from build123d import *

# Parameters (mm, degrees)
BOSS_EXTRUDE1_DEPTH                   = 6.35
FILLET1_R                             = 3.175
FILLET4_R                             = 0.508
F_1_4_0_25_DIAMETER_HOLE1_D           = 6.35
F_1_4_0_25_DIAMETER_HOLE1_ON_FACE_2_D = 6.35
FILLET8_R                             = 9.525


with BuildPart() as part:
    # Sketch1 → Boss-Extrude1 (new, symmetric)
    # profile 1 of 13: a face of its own
    with BuildSketch(Plane(origin=(0, 0, 0), x_dir=(1, 0, 0), z_dir=(0, 1, 0))):
        Polygon((-63.032869919, 6.829847883), (-50.8, 3.417093343), (-50.117449092, 5.863667327), (-48.008399772, 13.423462702), (-63.032869919, 17.128450878), align=None)
    # profile 2 of 13: a face of its own
    with BuildSketch(Plane(origin=(0, 0, 0), x_dir=(1, 0, 0), z_dir=(0, 1, 0))):
        with BuildLine():
            Line((-50.117449092, 5.863667327), (-50.8, 3.417093343))
            add(Edge.make_bspline(
                [(-50.8, 3.417093343), (-47.90401251, 2.638759622), (-42.323161066, 1.207315918), (-34.243320379, -0.564459364), (-28.828072067, -1.650873486), (-26.114874946, -2.164171794), (-25.868230414, -2.21056185)],
                knots=[0.402881469, 0.402881469, 0.402881469, 0.402881469, 0.417195876, 0.430379519, 0.442362633, 0.443560626, 0.443560626, 0.443560626, 0.443560626], degree=3))
            Line((-25.868230414, -2.21056185), (-25.529380555, -0.995969297))
            Line((-25.529380555, -0.995969297), (-50.117449092, 5.863667327))
        make_face()
    # profile 3 of 13: a face of its own
    with BuildSketch(Plane(origin=(0, 0, 0), x_dir=(1, 0, 0), z_dir=(0, 1, 0))):
        with BuildLine():
            add(Edge.make_bspline(
                [(-142.916964795, 26.637840254), (-139.851770269, 26.044031657), (-132.224118107, 24.507766264), (-120.204077857, 21.875031645), (-107.039843971, 18.731571582), (-94.42881917, 15.508074422), (-82.464130524, 12.283599717), (-72.07374601, 9.383281264), (-65.6770572, 7.577167824), (-63.032869919, 6.829847883)],
                knots=[0.2516695, 0.2516695, 0.2516695, 0.2516695, 0.266573311, 0.288810349, 0.310405036, 0.331177743, 0.350943876, 0.3695564, 0.382673151, 0.382673151, 0.382673151, 0.382673151], degree=3))
            Line((-63.032869919, 6.829847883), (-63.032869919, 17.128450878))
            Line((-63.032869919, 17.128450878), (-131.41505653, 33.991287994))
            ThreePointArc((-131.41505653, 33.991287994), (-135.697076354, 28.016927932), (-142.916964795, 26.637840254))
        make_face()
    # profile 4 of 13: a face of its own
    with BuildSketch(Plane(origin=(0, 0, 0), x_dir=(1, 0, 0), z_dir=(0, 1, 0))):
        with BuildLine():
            Line((-48.008399772, 13.423462702), (-50.117449092, 5.863667327))
            Line((-50.117449092, 5.863667327), (-25.529380555, -0.995969297))
            Line((-25.529380555, -0.995969297), (-21.592172885, 13.116780012))
            ThreePointArc((-21.592172885, 13.116780012), (-33.805570634, 3.783353047), (-46.135923457, 12.961715796))
            Line((-46.135923457, 12.961715796), (-48.008399772, 13.423462702))
        make_face()
    # profile 5 of 13: a face of its own
    with BuildSketch(Plane(origin=(0, 0, 0), x_dir=(1, 0, 0), z_dir=(0, 1, 0))):
        Polygon((-63.032869919, 20.214556587), (-63.032869919, 17.128450878), (-48.008399772, 13.423462702), (-46.180241275, 19.976417164), (-46.113804584, 20.214556587), align=None)
    # profile 6 of 13: a face of its own
    with BuildSketch(Plane(origin=(0, 0, 0), x_dir=(1, 0, 0), z_dir=(0, 1, 0))):
        with BuildLine():
            add(Edge.make_bspline(
                [(-152.4, 28.398178215), (-150.835767653, 28.120675984), (-147.672379647, 27.546477658), (-144.513670254, 26.947163992), (-142.916964795, 26.637840254)],
                knots=[0.236322429, 0.236322429, 0.236322429, 0.236322429, 0.243905882, 0.2516695, 0.2516695, 0.2516695, 0.2516695], degree=3))
            ThreePointArc((-142.916964795, 26.637840254), (-149.167660925, 30.710139705), (-150.804662589, 37.988535853))
            Line((-150.804662589, 37.988535853), (-152.4, 28.398178215))
        make_face()
    # profile 7 of 13: a face of its own
    with BuildSketch(Plane(origin=(0, 0, 0), x_dir=(1, 0, 0), z_dir=(0, 1, 0))):
        with BuildLine():
            ThreePointArc((-150.804662589, 37.988535853), (-149.167660925, 30.710139705), (-142.916964795, 26.637840254))
            ThreePointArc((-142.916964795, 26.637840254), (-135.697076354, 28.016927932), (-131.41505653, 33.991287994))
            ThreePointArc((-131.41505653, 33.991287994), (-131.199232943, 35.168440277), (-131.126940024, 36.363028513))
            ThreePointArc((-131.126940024, 36.363028513), (-138.72556699, 45.996556718), (-149.864041918, 40.850842606))
            ThreePointArc((-149.864041918, 40.850842606), (-150.443809774, 39.45565952), (-150.804662589, 37.988535853))
        make_face()
        with BuildLine():
            ThreePointArc((-136.206940024, 36.363028513), (-136.242159651, 35.781049629), (-136.347304475, 35.207565183))
            ThreePointArc((-136.347304475, 35.207565183), (-145.823720397, 36.945007397), (-136.206940024, 36.363028513))
        make_face(mode=Mode.SUBTRACT)
    # profile 8 of 13: a face of its own
    with BuildSketch(Plane(origin=(0, 0, 0), x_dir=(1, 0, 0), z_dir=(0, 1, 0))):
        with BuildLine():
            Line((-46.180241275, 19.976417164), (-48.008399772, 13.423462702))
            Line((-48.008399772, 13.423462702), (-46.135923457, 12.961715796))
            ThreePointArc((-46.135923457, 12.961715796), (-46.649452433, 16.465962078), (-46.180241275, 19.976417164))
        make_face()
    # profile 9 of 13: a face of its own
    with BuildSketch(Plane(origin=(0, 0, 0), x_dir=(1, 0, 0), z_dir=(0, 1, 0))):
        with BuildLine():
            Line((-152.4, 28.398178215), (-150.804662589, 37.988535853))
            Line((-150.804662589, 37.988535853), (-150.316016511, 40.926027704))
            Line((-150.316016511, 40.926027704), (-162.843866, 43.010011192))
            Line((-162.843866, 43.010011192), (-164.927849489, 30.482161703))
            add(Edge.make_bspline(
                [(-164.927849489, 30.482161703), (-163.914067431, 30.324847033), (-159.732455899, 29.664434578), (-155.558182899, 28.958454826), (-152.4, 28.398178215)],
                knots=[0.216114261, 0.216114261, 0.216114261, 0.216114261, 0.221011446, 0.236322429, 0.236322429, 0.236322429, 0.236322429], degree=3))
        make_face()
    # profile 10 of 13: a face of its own
    with BuildSketch(Plane(origin=(0, 0, 0), x_dir=(1, 0, 0), z_dir=(0, 1, 0))):
        with BuildLine():
            Line((-150.316016511, 40.926027704), (-150.804662589, 37.988535853))
            ThreePointArc((-150.804662589, 37.988535853), (-150.443809774, 39.45565952), (-149.864041918, 40.850842606))
            Line((-149.864041918, 40.850842606), (-150.316016511, 40.926027704))
        make_face()
    # profile 11 of 13: a face of its own
    with BuildSketch(Plane(origin=(0, 0, 0), x_dir=(1, 0, 0), z_dir=(0, 1, 0))):
        with BuildLine():
            Line((-164.927849489, 30.482161703), (-152.4, 28.398178215))
            add(Edge.make_bspline(
                [(-164.927849489, 30.482161703), (-163.914067431, 30.324847033), (-159.732455899, 29.664434578), (-155.558182899, 28.958454826), (-152.4, 28.398178215)],
                knots=[0.216114261, 0.216114261, 0.216114261, 0.216114261, 0.221011446, 0.236322429, 0.236322429, 0.236322429, 0.236322429], degree=3))
        make_face()
    # profile 12 of 13: a face of its own
    with BuildSketch(Plane(origin=(0, 0, 0), x_dir=(1, 0, 0), z_dir=(0, 1, 0))):
        with BuildLine():
            Line((-46.113804584, 20.214556587), (-46.180241275, 19.976417164))
            ThreePointArc((-46.180241275, 19.976417164), (-46.14635129, 20.095654256), (-46.111304881, 20.214556587))
            Line((-46.111304881, 20.214556587), (-46.113804584, 20.214556587))
        make_face()
    # profile 13 of 13: a face of its own
    with BuildSketch(Plane(origin=(0, 0, 0), x_dir=(1, 0, 0), z_dir=(0, 1, 0))):
        with BuildLine():
            ThreePointArc((-46.111304881, 20.214556587), (-46.14635129, 20.095654256), (-46.180241275, 19.976417164))
            ThreePointArc((-46.180241275, 19.976417164), (-46.649452433, 16.465962078), (-46.135923457, 12.961715796))
            ThreePointArc((-46.135923457, 12.961715796), (-33.805570634, 3.783353047), (-21.592172885, 13.116780012))
            ThreePointArc((-21.592172885, 13.116780012), (-21.240618227, 14.815698867), (-21.122707154, 16.546598324))
            ThreePointArc((-21.122707154, 16.546598324), (-32.032575932, 29.17478044), (-46.111304881, 20.214556587))
        make_face()
        with BuildLine():
            ThreePointArc((-27.472707154, 16.546598324), (-29.931164004, 11.497775102), (-35.421757105, 10.319635293))
            ThreePointArc((-35.421757105, 10.319635293), (-37.841250304, 21.595421547), (-27.472707154, 16.546598324))
        make_face(mode=Mode.SUBTRACT)
    extrude(amount=BOSS_EXTRUDE1_DEPTH, both=True)

    # Fillet1
    # the kernel refuses this fillet: 3.175 mm, written as the material it adds along each edge
    with BuildSketch(Plane(origin=(-149.864041918, 6.35, -40.850842606), x_dir=(0.5331827682272952, 0, -0.8460000801805391), z_dir=(0, -1, 0))) as fillet1_piece_1:
        with BuildLine():
            CenterArc((2.116076272, -3.161518606), FILLET1_R, 95.281860793, 61.941944222)
            Line((-0.811350167, -1.932372788), (0, 0))
            ThreePointArc((0, 0), (0.911900272, -0.042061948), (1.823800544, 0))
        make_face()
    extrude(amount=12.7)
    with BuildSketch(Plane(origin=(-131.41505653, -6.35, -33.991287994), x_dir=(0.9709149499625199, 0, 0.23942464355048618), z_dir=(0, 1, 0))) as fillet1_piece_2:
        with BuildLine():
            CenterArc((2.783835933, 3.175), FILLET1_R, 194.047041006, 75.952958994)
            ThreePointArc((-0.296221332, 2.404368932), (-0.074334234, 1.211273817), (0, 0))
            Line((0, 0), (2.783835933, 0))
        make_face()
    extrude(amount=12.7)
    with BuildSketch(Plane(origin=(-46.111304881, 6.35, -20.214556587), x_dir=(-1, 0, 0), z_dir=(0, -1, 0)), Plane(origin=(-46.111304881, 0, -20.214556587), x_dir=(-1, 0, 0), z_dir=(0, -1, 0))) as fillet1_piece_3:
        with BuildLine():
            CenterArc((2.169682732, 3.175), FILLET1_R, 205.425374389, 64.574625611)
            ThreePointArc((-0.697803415, 1.811860904), (-0.314399096, 0.91921847), (0, 0))
            Line((0, 0), (2.169682732, 0))
        make_face()
    extrude(amount=6.35)
    # the kernel refuses this fillet: 3.175 mm, written as the material it takes off along each edge
    with BuildSketch(Plane(origin=(-162.843866, 14.2875, -43.010011192), x_dir=(-0.16409318808875556, 0, 0.9864448416525216), z_dir=(0, -1, 0))) as fillet1_2_piece_1:
        with BuildLine():
            CenterArc((FILLET1_R, -FILLET1_R), FILLET1_R, 90, 90)
            Line((0, -FILLET1_R), (0, 0))
            Line((0, 0), (FILLET1_R, 0))
        make_face()
    extrude(amount=28.575, mode=Mode.SUBTRACT)

    # Fillet4
    fillet4_edges = [part.edges().sort_by_distance(p)[0] for p in [
        (-164.927849489, 0, -30.482161703),
        (-63.032869919, 0, -17.128450878),
        (-63.032869919, 0, -20.214556587),
    ]]
    fillet(fillet4_edges, radius=FILLET4_R)

    # 1/4 (0.25) Diameter Hole1 (through all)
    with Locations(Plane(origin=(-56.916434959, 0, -5.123470613), x_dir=(0.963218103856, 0, 0.268720829868), z_dir=(-0.268720829868, 0, 0.963218103856))):
        with Locations((0, 0)):
            Hole(F_1_4_0_25_DIAMETER_HOLE1_D / 2)

    # 1/4 (0.25) Diameter Hole1 on face 2 (through all)
    with Locations(Plane(origin=(-158.663924744, 0, -29.440169959), x_dir=(0.986444876362, 0, 0.164092979433), z_dir=(-0.164092979433, 0, 0.986444876362))):
        with Locations((0, 0)):
            Hole(F_1_4_0_25_DIAMETER_HOLE1_ON_FACE_2_D / 2)

    # Fillet8
    fillet8_edges = [part.edges().sort_by_distance(p)[0] for p in [
        (-25.868230414, -3.175, 2.21056185),
    ]]
    fillet(fillet8_edges, radius=FILLET8_R)


solid = part.part
Verification items for the finished model (mm, model axes). A direction names the side the tool comes from. Give positions to 0.01 mm unless a question says otherwise; leave off trailing zeros.
(1) Gauge pin test, flat ends, axial feed: pin 1 (2 mm diameter, centred on y = 1, z = -23.5, fed in from +X); pin 2 (6.5 mm diameter, centred on x = -54.5, y = -3, fed in from -Z); pin 3 (1 mm diameter, centred on x = -121, y = 0, fed in from +Z); pin 4 (7.5 mm diameter, centred on x = -141.03, z = -36.36, fed in from -Y). Record the tip position at first contact, or that the pin passes through.
(2) Material ranges on line 1 (X direction, y = -2.75, z = -35); line 2 (X direction, y = -5.5, z = -39); line 3 (Z direction, x = -140, y = 5.5), recorded low to high.
(3) Mould release check, pull along Z, two halves, no side actions. Record for faces 3 (the face through (-95.73, -0.09, -25.19)), 4 (the face through (-136.575, -0.089, -38.211)), 5 (the face through (-155.825, -2.911, -28.968)): +Z half, -Z half, draft (parallel to the pull), parting line (faces both ways), or undercut.
(4) Access from +Z, -Z, +X, -X, +Y, -Y to the whole of each face (thin tool, end or side, straight path). Record for faces 1 (the face through (-57, 0, -20.215)), 2 (the face through (-27.96, -0.09, -19)).
(5) Cross-section at A-A (y = -1.75). State how many separate pieces and enclosed holes the cut face has, plus the area to 3 significant figures.
Worked out:
1. pin 1: stops at x = -22.6
1. pin 2: stops at z = -20.21
1. pin 3: stops at z = -21.9
1. pin 4: passes through
2. line 1: x = -164.18 to -159.35, -156.13 to -145.66, -136.4 to -130.8
2. line 2: x = -163.51 to -145.07, -136.99 to -131.48
2. line 3: z = -46.22 to -41.08, -31.65 to -26.07
3. face 3: -Z half
3. face 4: undercut
3. face 5: +Z half
4. face 1: -Z, +Y, -Y
4. face 2: +Y, -Y
5. separate pieces: 3
5. enclosed holes: 2
5. area: 1,710 mm2
